```python
from build123d import *

# Parameters (mm, degrees)
CROQUIS1_W              = 200
CROQUIS1_H              = 300
SALIENTE_EXTRUIR1_DEPTH = 5
CROQUIS2_W              = 60
CROQUIS2_H              = 5
CORTAR_EXTRUIR1_DEPTH   = 181.346887969
EXTRUIR_L_MINA1_DEPTH   = 200
CROQUIS7_W              = 190
CROQUIS7_H              = 272.300046581
CORTAR_EXTRUIR2_DEPTH   = 183.756668825


with BuildPart() as part:
    # Croquis1 → Saliente-Extruir1 (new body)
    with BuildSketch(Plane.XY):
        Rectangle(CROQUIS1_W, CROQUIS1_H)
    extrude(amount=SALIENTE_EXTRUIR1_DEPTH)

    # Croquis2 → Cortar-Extruir1 (cut, through all)
    with BuildSketch(Plane.XY.offset(5)):
        with Locations((-55, 107.5)):
            Rectangle(CROQUIS2_W, CROQUIS2_H)
        with Locations((55, 107.5)):
            Rectangle(CROQUIS2_W, CROQUIS2_H)
        with Locations((55, 90.961538462)):
            Rectangle(CROQUIS2_W, CROQUIS2_H)
        with Locations((55, 74.423076923)):
            Rectangle(CROQUIS2_W, CROQUIS2_H)
        with Locations((55, 57.884615385)):
            Rectangle(CROQUIS2_W, CROQUIS2_H)
        with Locations((55, 41.346153846)):
            Rectangle(CROQUIS2_W, CROQUIS2_H)
        with Locations((55, 24.807692308)):
            Rectangle(CROQUIS2_W, CROQUIS2_H)
        with Locations((55, 8.269230769)):
            Rectangle(CROQUIS2_W, CROQUIS2_H)
        with Locations((55, -8.269230769)):
            Rectangle(CROQUIS2_W, CROQUIS2_H)
        with Locations((55, -24.807692308)):
            Rectangle(CROQUIS2_W, CROQUIS2_H)
        with Locations((55, -41.346153846)):
            Rectangle(CROQUIS2_W, CROQUIS2_H)
        with Locations((55, -57.884615385)):
            Rectangle(CROQUIS2_W, CROQUIS2_H)
        with Locations((55, -74.423076923)):
            Rectangle(CROQUIS2_W, CROQUIS2_H)
        with Locations((55, -90.961538462)):
            Rectangle(CROQUIS2_W, CROQUIS2_H)
        with Locations((55, -107.5)):
            Rectangle(CROQUIS2_W, CROQUIS2_H)
        with Locations((-55, 90.961538462)):
            Rectangle(CROQUIS2_W, CROQUIS2_H)
        with Locations((-55, 74.423076923)):
            Rectangle(CROQUIS2_W, CROQUIS2_H)
        with Locations((-55, 57.884615385)):
            Rectangle(CROQUIS2_W, CROQUIS2_H)
        with Locations((-55, 41.346153846)):
            Rectangle(CROQUIS2_W, CROQUIS2_H)
        with Locations((-55, 24.807692308)):
            Rectangle(CROQUIS2_W, CROQUIS2_H)
        with Locations((-55, 8.269230769)):
            Rectangle(CROQUIS2_W, CROQUIS2_H)
        with Locations((-55, -8.269230769)):
            Rectangle(CROQUIS2_W, CROQUIS2_H)
        with Locations((-55, -24.807692308)):
            Rectangle(CROQUIS2_W, CROQUIS2_H)
        with Locations((-55, -41.346153846)):
            Rectangle(CROQUIS2_W, CROQUIS2_H)
        with Locations((-55, -57.884615385)):
            Rectangle(CROQUIS2_W, CROQUIS2_H)
        with Locations((-55, -74.423076923)):
            Rectangle(CROQUIS2_W, CROQUIS2_H)
        with Locations((-55, -90.961538462)):
            Rectangle(CROQUIS2_W, CROQUIS2_H)
        with Locations((-55, -107.5)):
            Rectangle(CROQUIS2_W, CROQUIS2_H)
    extrude(amount=-CORTAR_EXTRUIR1_DEPTH, mode=Mode.SUBTRACT)

    # Croquis5 → Extruir-Lámina1 (add)
    with BuildSketch(Plane.ZY.offset(100)):
        with BuildLine():
            Line((5, 85), (17.5, 85))
            ThreePointArc((17.5, 85), (30, 97.5), (17.5, 110))
            Line((17.5, 110), (5, 110))
            Line((5, 110), (5, 115))
            Line((5, 115), (17.5, 115))
            ThreePointArc((17.5, 115), (35, 97.5), (17.5, 80))
            Line((17.5, 80), (5, 80))
            Line((5, 80), (5, 85))
        make_face()
        with BuildLine():
            Line((5, -110), (17.5, -110))
            ThreePointArc((17.5, -110), (30, -97.5), (17.5, -85))
            Line((17.5, -85), (5, -85))
            Line((5, -85), (5, -80))
            Line((5, -80), (17.5, -80))
            ThreePointArc((17.5, -80), (35, -97.5), (17.5, -115))
            Line((17.5, -115), (5, -115))
            Line((5, -115), (5, -110))
        make_face()
    extrude(amount=-EXTRUIR_L_MINA1_DEPTH)

    # Croquis7 → Cortar-Extruir2 (cut, through all)
    with BuildSketch(Plane.XY.offset(5)):
        with Locations((0, 8.640872113)):
            Rectangle(CROQUIS7_W, CROQUIS7_H)
    extrude(amount=CORTAR_EXTRUIR2_DEPTH, mode=Mode.SUBTRACT)


solid = part.part
```
Verification items for the finished model (mm, model axes). A direction names the side the tool comes from. Give positions to 0.01 mm unless a question says otherwise; leave off trailing zeros. Loops run counter-clockwise (first coordinate to the right, second up) from the corner with the lowest first, then second, coordinate; pieces in that order, holes last.
1. Mould release check, pull along X, two halves, no side actions. Record for faces 1 (the flat face through (95, -100, 30)), 2 (the flat face through (100, 0.7, 4.6)), 3 (the cylindrical face through (-97.535, -97.115, 34.996)): released by +X, released by -X, zero draft, split by the parting line, or undercut.
2. Thickness scan on line 1 (Z direction, x = 26.5, y = -94); line 2 (X direction, y = -83, z = 22.5). Record the ranges inside material, lowest first.
3. Section check B-B, the plane y = 97.5. Enter the section's corners in (x, z), then the cut area to 3 significant figures.
4. Section check A-A, the plane z = 9. Count the separate pieces of the cut face and the enclosed holes in it, then the cut area to 3 significant figures.
5. Set-up check for faces 4 (the flat face through (-95, 95, 30)), 5 (the cylindrical face through (-97.535, 97.225, 29.997)), 6 (the cylindrical face through (-97.535, 97.885, 34.996)): record each of +Z, -Z, +X, -X, +Y, -Y from which the full face is reachable in a straight line by a thin tool's end or side.
6. Go/stop test with flat-tipped pins: pin 1 Ø5.5 at (x, z) = (98.5, 12.5) entering from -Y; pin 2 Ø5 at (x, y) = (-16, -86.5) entering from +Z; pin 3 Ø4 at (x, y) = (-10.5, -33) entering from -Z; pin 4 Ø4 at (x, z) = (96.5, 13) entering from +Y. Record where each tip stops, or that it passes through.
Geometry says:
1. face 1: undercut
1. face 2: released by +X
1. face 3: zero draft
2. line 1: z = 0 to 5
2. line 2: x = -100 to -95, 95 to 100
3. outline: (-100, 0) - (100, 0) - (100, 5) - (-100, 5) - close; (-100, 30) - (-95, 30) - (-95, 35) - (-100, 35) - close; (95, 30) - (100, 30) - (100, 35) - (95, 35) - close
3. area: 1,050 mm2
4. separate pieces: 8
4. enclosed holes: 0
4. area: 200 mm2
5. face 4: +Z, +Y, -Y
5. face 5: +X, -X
5. face 6: +Z, +X, -X
6. pin 1: stops at y = -115
6. pin 2: stops at z = 5
6. pin 3: stops at z = 0
6. pin 4: stops at y = 115
